Verification items for the finished model (mm, model axes). A direction names the side the tool comes from. Give positions to 0.01 mm unless a question says otherwise; leave off trailing zeros. Write each loop counter-clockwise with the first axis right and the second up, starting at its lowest first coordinate (ties: lowest second). Pieces come first, ordered by that corner, then holes. Notation, with made-up numbers: M -32,82.25 L -18,82.25 A23 cw -18,106.25 Z; hole C 51.5,43 d1. An arc over 180 degrees is marked long. Answer as a JSON object with one key per item and string values.
Autodesk Inventor part; units mm, degrees
ref_plane "YZ Plane" through (0, 0, 0) normal (1, 0, 0) x (0, 1, 0)
ref_plane "XZ Plane" through (0, 0, 0) normal (0, 1, 0) x (-1, 0, 0)
ref_plane "XY Plane" through (0, 0, 0) normal (0, 0, 1) x (1, 0, 0)
sketch "Sketch1" plane through (0, 0, 0) normal (0, 1, 0) x (-1, 0, 0)
  line L0 (60, 0) -> (60, -1)
  line L1 (1, -60) -> (0, -60)
  line L2 (0, 0) -> (0, -40)
  line L3 (1, -1) -> (1, -40)
  line L4 (1, -40) -> (0, -40)
  line L5 (0, 0) -> (40, 0)
  line L6 (1, -1) -> (40, -1)
  line L7 (40, -1) -> (40, 0)
  dimension "d0" = 60
  dimension "d2" = 1
  dimension "d15" = 40
  dimension "d24" = 40
extrude "Extrusion1" add sketch "Sketch1" along normal blind 60
fillet "Fillet1" radius 2 1 edges at (0, 30, 0)
sketch "Sketch4" plane through (0, 0, -40) normal (1, 0, 0) x (0, 0, -1)
  circle A0 centre (-10, 40) radius 1.5
  circle A1 centre (-10, 20) radius 1.5
  point P0 (-40, 0)
  dimension "d17" = 3
  dimension "d18" = 3
extrude "Extrusion4" cut sketch "Sketch4" against normal blind 1
sketch "Sketch5" plane through (-40, 0, 0) normal (0, 0, 1) x (1, 0, 0)
  circle A0 centre (10, 40) radius 1.5
  circle A1 centre (10, 20) radius 1.5
  point P0 (40, 0)
  dimension "d25" = 3
  dimension "d27" = 3
extrude "Extrusion5" cut sketch "Sketch5" against normal blind 1
properties part number "clamp"
1) Section check A-A on x = -30. Record the boundary of the cut face in (y, z).
Completed:
{"outline": "M 0,-1 L 18.5,-1 L 18.5,0 L 0,0 Z; M 21.5,-1 L 38.5,-1 L 38.5,0 L 21.5,0 Z; M 41.5,-1 L 60,-1 L 60,0 L 41.5,0 Z"}
2) Release check for a two-part mould opening along Y. For faces 1 (the face through (-0.5, 39.1, -28.8)), 2 (the face through (-1, 30, -20)), 3 (the face through (-11, 0, -0.6)), 4 (the face through (-31.11, 21.01, -0.49)) record: pulls with the +Y half, pulls with the -Y half, needs draft (parallel to the pull), parting line crosses it, or undercut.
Completed:
{"face 1": "undercut", "face 2": "needs draft", "face 3": "pulls with the -Y half", "face 4": "undercut"}
3) Access from +Z, -Z, +X, -X, +Y, -Y to the whole of each face (thin tool, end or side, straight path). Record for faces 5 (the face through (-0.49, 21.01, -28.89)), 6 (the face through (-20, 30, -1)).
Completed:
{"face 5": "+X, -X", "face 6": "-Z, -X, +Y, -Y"}
4) Section check B-B on y = 20. Record the boundary of the cut face in (x, z).
Completed:
{"outline": "M -40,-1 L -31.5,-1 L -31.5,0 L -40,0 Z; M -28.5,-1 L -1,-1 L -1,-28.5 L 0,-28.5 L 0,-2 A2 ccw -2,0 L -28.5,0 Z; M -1,-40 L 0,-40 L 0,-31.5 L -1,-31.5 Z"}
5) Section check D-D on y = 11. Record the boundary of the cut face in (x, z).
Completed:
{"outline": "M -40,-1 L -1,-1 L -1,-40 L 0,-40 L 0,-2 A2 ccw -2,0 L -40,0 Z"}
6) Go/stop test with flat-tipped pins: pin 1 (10 mm diameter, centred on y = 9, z = -14.5, fed in from +X); pin 2 (6 mm diameter, centred on x = -33, y = 46.5, fed in from -Z); pin 3 (4 mm diameter, centred on y = 20, z = -30, fed in from -X). Record where each tip stops, or that it passes through.
Completed:
{"pin 1": "stops at x = 0", "pin 2": "stops at z = -1", "pin 3": "stops at x = -1"}
7) Thickness scan on L1, parallel to Y at x = -0.55, z = -30; L2, parallel to Z at x = -22, y = 23.5. Record the ranges inside material, lowest first.
Completed:
{"L1": "y = 0 to 18.5, 21.5 to 38.5, 41.5 to 60", "L2": "z = -1 to 0"}
8) Section check C-C on z = -30. Record the boundary of the cut face in (x, y).
Completed:
{"outline": "M -1,0 L 0,0 L 0,18.5 L -1,18.5 Z; M -1,21.5 L 0,21.5 L 0,38.5 L -1,38.5 Z; M -1,41.5 L 0,41.5 L 0,60 L -1,60 Z"}
